Autodesk Inventor part; units mm, degrees
ref_plane "YZ Plane" through (0, 0, 0) normal (1, 0, 0) x (0, 1, 0)
ref_plane "XZ Plane" through (0, 0, 0) normal (0, 1, 0) x (-1, 0, 0)
ref_plane "XY Plane" through (0, 0, 0) normal (0, 0, 1) x (1, 0, 0)
sketch "Sketch1" plane through (0, 0, 0) normal (1, 0, 0) x (0, 1, 0)
  line L0 (73.575, 28) -> (65.075, 28)
  line L1 (-73.575, 60) -> (-73.575, -60)
  line L2 (73.575, -28) -> (73.575, 28)
  circle A0 centre (59.575, 0) radius 4
  circle A1 centre (-12.425, 0) radius 4
  circle A2 centre (-46.575, 0) radius 5
  circle A3 centre (-46.575, 18.25) radius 2.5
  circle A4 centre (-46.575, -18.25) radius 2.5
  circle A5 centre (59.575, 0) radius 7.5
  line L3 (65.075, 28) -> (65.075, 5.099)
  line L4 (65.075, -5.099) -> (65.075, -28)
  circle A6 centre (51.575, -100) radius 4
  circle A7 centre (51.575, 100) radius 4
  arc A8 (65.075, 100) -> (46.1655, 112.3688) centre (51.575, 100) ccw
  arc A9 (46.1655, -112.3688) -> (65.075, -100) centre (51.575, -100) ccw
  line L5 (65.075, 28) -> (65.075, 100)
  line L6 (65.075, -28) -> (65.075, -100)
  line L7 (46.1655, 112.3688) -> (-73.575, 60)
  line L8 (-73.575, -60) -> (46.1655, -112.3688)
  line L9 (65.075, -28) -> (73.575, -28)
  line L10 (30.0644, 90.0466) -> (-40.7048, 59.0955)
  line L11 (30.0644, -90.0466) -> (-40.7048, -59.0955)
  line L12 (51.075, 76.3035) -> (51.075, 35)
  line L13 (51.075, -76.3035) -> (51.075, -35)
  line L14 (41.075, 25) -> (-33.575, 25)
  line L15 (41.075, -25) -> (-33.575, -25)
  arc A10 (41.075, 25) -> (51.075, 35) centre (41.075, 35) ccw
  arc A11 (-40.7048, 59.0955) -> (-33.575, 25) centre (-33.575, 42.7932) ccw
  arc A12 (51.075, -35) -> (41.075, -25) centre (41.075, -35) ccw
  line L16 (-31.8814, -25) -> (-33.575, -25)
  arc A13 (-33.575, -25) -> (-40.7048, -59.0955) centre (-33.575, -42.7932) ccw
  line L17 (1.575, 5) -> (1.575, -5)
  arc A14 (43.575, 5) -> (33.575, 15) centre (33.575, 5) ccw
  arc A15 (33.575, -15) -> (43.575, -5) centre (33.575, -5) ccw
  arc A16 (11.575, 15) -> (1.575, 5) centre (11.575, 5) ccw
  arc A17 (1.575, -5) -> (11.575, -15) centre (11.575, -5) ccw
  circle A18 centre (-61.575, 51.0593) radius 4
  circle A19 centre (-61.575, -51.0593) radius 4
  arc A20 (51.075, 76.3035) -> (30.0644, 90.0466) centre (36.075, 76.3035) ccw
  arc A21 (30.0644, -90.0466) -> (51.075, -76.3035) centre (36.075, -76.3035) ccw
  line L18 (43.575, 5) -> (43.575, -5)
  line L19 (33.575, 15) -> (11.575, 15)
  line L20 (33.575, -15) -> (11.575, -15)
  circle A22 centre (-20.425, 30) radius 4
  circle A23 centre (-20.425, 30) radius 12.5
  point P0 (0, 0)
  point P1 (73.575, 0)
  point P2 (51.075, 58.5072)
  point P3 (51.075, -58.5072)
  point P4 (-20.425, -42.5)
  point P5 (16.0532, -25)
  point P6 (-49.2726, -25)
  point P7 (51.075, 59.4738)
  point P8 (43.575, 0)
  point P9 (1.575, 0)
  dimension "d1" = 56
  dimension "d2" = 72
  dimension "d3" = 8
  dimension "d4" = 8
  dimension "d5" = 14
  dimension "d6" = 34.15
  dimension "d7" = 10
  dimension "d8" = 18.25
  dimension "d9" = 18.25
  dimension "d10" = 5
  dimension "d13" = 12.425
  dimension "d14" = 27
  dimension "d15" = 15
  dimension "d18" = 5.5
  dimension "d19" = 8
  dimension "d20" = 100
  dimension "d21" = 100
  dimension "d22" = 8
  dimension "d27" = 60
  dimension "d28" = 60
  dimension "d31" = 14
  dimension "d33" = 14
  dimension "d34" = 14
  dimension "d36" = 25
  dimension "d37" = 25
  dimension "d43" = 40
  dimension "d45" = 14
  dimension "d47" = 12
  dimension "d48" = 13
  dimension "d49" = 13
  dimension "d50" = 12
  dimension "d58" = 10
  dimension "d59" = 15
  dimension "d60" = 16
  dimension "d61" = 10
  dimension "d62" = 10
  dimension "d90" = 8
  dimension "d91" = 25
  dimension "d92" = 30
  dimension "d93" = 8
extrude "Extrusion3" add sketch "Sketch1" along normal blind 10 contours L3 A5 L4 L6 A9 L8 L1 L7 A8 L5 | A5 | A23 L14 | L14 A23
fillet "Fillet1" radius 6 3 edges at (5, -33.575, -25) (5, -31.8814, 25) (5, -8.9686, 25)
sketch "Sketch3" plane through (10, 0, 0) normal (1, 0, 0) x (0, 0, -1)
  line L0 (-18, -36.575) -> (18, -36.575)
  line L1 (18, -36.575) -> (18, -6)
  line L2 (18, -6) -> (-18, -6)
  line L3 (-18, -6) -> (-18, -36.575)
  line L4 (-15, 11.575) -> (-15, 33.575)
  line L5 (15, 33.575) -> (15, 11.575)
  circle A0 centre (0, -46.575) radius 5
  line L6 (-32.0593, -56.575) -> (32.0593, -56.575)
  line L7 (32.0593, -56.575) -> (32.0593, -68.575)
  line L8 (32.0593, -68.575) -> (-32.0593, -68.575)
  line L9 (-32.0593, -68.575) -> (-32.0593, -56.575)
  line L10 (-60, -73.575) -> (60, -73.575)
  line L11 (-102.0122, 29.9722) -> (-70.0199, -43.1778)
  line L12 (-94.6826, 33.1778) -> (-62.6903, -39.9722)
  line L13 (62.6903, -39.9722) -> (94.6826, 33.1778)
  line L14 (90.0466, 30.0644) -> (59.0955, -40.7048)
  line L15 (102.0122, 29.9722) -> (70.0199, -43.1778)
  line L16 (60, -73.575) -> (112.3688, 46.1655)
  arc A1 (-94.6826, 33.1778) -> (-102.0122, 29.9722) centre (-98.3474, 31.575) ccw
  arc A2 (-70.0199, -43.1778) -> (-62.6903, -39.9722) centre (-66.3551, -41.575) ccw
  arc A3 (102.0122, 29.9722) -> (94.6826, 33.1778) centre (98.3474, 31.575) ccw
  arc A4 (62.6903, -39.9722) -> (70.0199, -43.1778) centre (66.3551, -41.575) ccw
  line L17 (-59.0955, -40.7048) -> (-90.0466, 30.0644)
  line L18 (-112.3688, 46.1655) -> (-60, -73.575)
  line L19 (-80, 62.075) -> (-20, 62.075)
  line L20 (-20, 54.075) -> (-80, 54.075)
  line L21 (20, 62.075) -> (80, 62.075)
  line L22 (80, 54.075) -> (20, 54.075)
  arc A5 (-80, 62.075) -> (-80, 54.075) centre (-80, 58.075) ccw
  arc A6 (-20, 54.075) -> (-20, 62.075) centre (-20, 58.075) ccw
  arc A7 (20, 62.075) -> (20, 54.075) centre (20, 58.075) ccw
  arc A8 (80, 54.075) -> (80, 62.075) centre (80, 58.075) ccw
  circle A9 centre (0, 59.575) radius 4
  line L23 (-5.099, 65.075) -> (-100, 65.075)
  line L24 (-76.3035, 51.075) -> (-35, 51.075)
  line L25 (35, 51.075) -> (76.3035, 51.075)
  line L26 (100, 65.075) -> (5.099, 65.075)
  circle A10 centre (0, -12.425) radius 7
  circle A11 centre (0, -12.425) radius 4
  circle A12 centre (-100, 51.575) radius 4
  circle A13 centre (100, 51.575) radius 4
  circle A14 centre (-51.0593, -61.575) radius 4
  circle A15 centre (-51.0593, -61.575) radius 4
  circle A16 centre (-100, 51.575) radius 4
  circle A17 centre (100, 51.575) radius 4
  circle A18 centre (-51.0593, -61.575) radius 4
  point P0 (0, 0)
  dimension "d63" = 3
  dimension "d64" = 3
  dimension "d65" = 6
  dimension "d66" = 10
  dimension "d67" = 5
  dimension "d68" = 10
  dimension "d71" = 3
  dimension "d72" = 3
  dimension "d73" = 3
  dimension "d74" = 3
  dimension "d78" = 20
  dimension "d79" = 20
  dimension "d81" = 3
  dimension "d82" = 3
  dimension "d83" = 3
  dimension "d84" = 3
  dimension "d87" = 14
  dimension "d113" = 20
  dimension "d114" = 20
  dimension "d115" = 20
  dimension "d117" = 20
extrude "Extrusion5" cut sketch "Sketch3" against normal blind 5 contours L3 L2 A10 L1 L0 | L6 L7 L8 L9 | A1 L12 A2 L11 | L13 A3 L15 A4 | L19 A6 L20 A5 | L21 A8 L22 A7
fillet "Fillet2" radius 4 10 edges at (7.5, -6, 18) (7.5, -36.575, 18) (7.5, -36.575, -18) (7.5, -6, -18) (7.5, -6, 2.7784) (7.5, -6, -2.7784) (7.5, -56.575, 32.0593) (7.5, -56.575, -32.0593) (7.5, -68.575, -32.0593) (7.5, -68.575, 32.0593)
sketch "Sketch4" plane through (10, -32.6529, 0.9304) normal (1, 0, 0) x (0, 0, -1)
  circle A0 centre (-9.0696, 92.2279) radius 1.5
  circle A1 centre (10.9304, 92.2279) radius 1.5
  circle A2 centre (0.9304, 92.2279) radius 4
  circle A3 centre (0.9304, 92.2279) radius 4
  circle A4 centre (0.9304, 92.2279) radius 4
  circle A5 centre (-9.0696, 20.2279) radius 1.5
  circle A6 centre (10.9304, 20.2279) radius 1.5
  circle A7 centre (0.9304, 20.2279) radius 4
  circle A8 centre (0.9304, 20.2279) radius 4
  circle A9 centre (0.9304, 20.2279) radius 4
  circle A10 centre (0.9304, 20.2279) radius 4
  circle A11 centre (-9.0696, 20.2279) radius 1.5
  circle A12 centre (10.9304, 20.2279) radius 1.5
  point P0 (0, 0)
  dimension "d106" = 3
  dimension "d105" = 10
  dimension "d104" = 10
  dimension "d110" = 3
  dimension "d111" = 10
  dimension "d112" = 10
extrude "Extrusion6" cut sketch "Sketch4" against normal blind 10 contours A0 | A1 | A5 | A6
properties part number "Frame_Bearing"
Design review of the part built by this model. Coordinates are the model's own, in mm. A direction names the side the tool comes from. Coordinates: 2 decimals unless noted, no trailing zeros. Loops run counter-clockwise (first coordinate to the right, second up) from the corner with the lowest first, then second, coordinate; pieces in that order, holes last. Notation, with made-up numbers: (71.25, 21) -> (125.25, 21) arc R3 ccw to (125.25, 26) -> close; hole circle Ø7 at (-31, -18.5). An arc over 180 degrees is marked (long way). Use a Markdown table: item, result. Add a question column.
Item 1: Clearance check with flat-ended pins moving along their axes: P1, Ø6, axis at x = 8.5, y = -50, coming from the -Z side; P2, Ø3, axis at x = 4.5, z = -43, coming from the +Y side (3 decimals); P3, Ø5, axis at x = 5.5, y = 26, coming from the -Z side; P4, Ø6.5, axis at y = 51.575, z = -100, coming from the +X side. State where each tip first meets the part, or that it passes through.
Item 2: We need section B-B, the plane x = 7. Count the separate pieces of the cut face and the enclosed holes in it, and give its area (3 significant figures).
Item 3: We need section A-A, the plane y = -22. Write out the cut boundary in (x, z).
Item 4: Wall thickness on L1, parallel to Z at x = 7.25, y = 22; L2, parallel to Z at x = 2.75, y = 4.5; L3, parallel to Y at x = 3.5, z = 10 (3 decimals): over which ranges is each line inside the solid? List them lowest first. Write a range as from..to.
Item 5: Machinability: for faces 4 (the cylindrical face through (7.465, -7.542, -7.574)), 5 (the flat face through (5, 1.575, 0)), which of the approach directions +Z, -Z, +X, -X, +Y, -Y give a long, thin tool a straight path to every point of the face, cutting with its end or side? Answer none if there is none.
Item 6: The part is to be moulded in two halves that separate along Z. For faces 1 (the flat face through (5, 65.075, -52)), 2 (the flat face through (4.93, -12.87, 86.55)), 3 (the cylindrical face through (8, 58, -84)), say which applies: +Z half, -Z half, draft (parallel to the pull), parting line (faces both ways), or undercut.
Numbers:
| question | item | result |
|---|---|---|
| 1 | P1 | stops at z = -71.62 |
| 1 | P2 | stops at y = 65.075 |
| 1 | P3 | stops at z = -104.64 |
| 1 | P4 | passes through |
| 2 | separate pieces | 1 |
| 2 | enclosed holes | 21 |
| 2 | area | 9,330 mm^2 |
| 3 | outline | (0, -82.56) -> (10, -82.56) -> (10, -79.28) -> (5, -79.28) -> (5, -70.55) -> (10, -70.55) -> (10, -67.28) -> (0, -67.28) -> close; (0, -25) -> (10, -25) -> (10, -18) -> (5, -18) -> (5, 18) -> (10, 18) -> (10, 26.32) -> (0, 26.32) -> close; (0, 33.68) -> (10, 33.68) -> (10, 42.4) -> (0, 42.4) -> close; (0, 67.28) -> (10, 67.28) -> (10, 70.55) -> (5, 70.55) -> (5, 79.28) -> (10, 79.28) -> (10, 82.56) -> (0, 82.56) -> close |
| 4 | L1 | z = -101.8..-98.53, -89.79..-86.52, -25..-15, 15..25, 86.52..89.79, 98.53..101.8 |
| 4 | L2 | z = -94.15..-78.87, -25..-12.07, 12.07..25, 78.87..94.15 |
| 4 | L3 | y = -73.575..-13.925, -10.925..2.915, 42.235..58.075, 61.075..65.075 |
| 5 | face 4 | +X |
| 5 | face 5 | +X, -X |
| 6 | face 1 | draft |
| 6 | face 2 | +Z half |
| 6 | face 3 | undercut |
